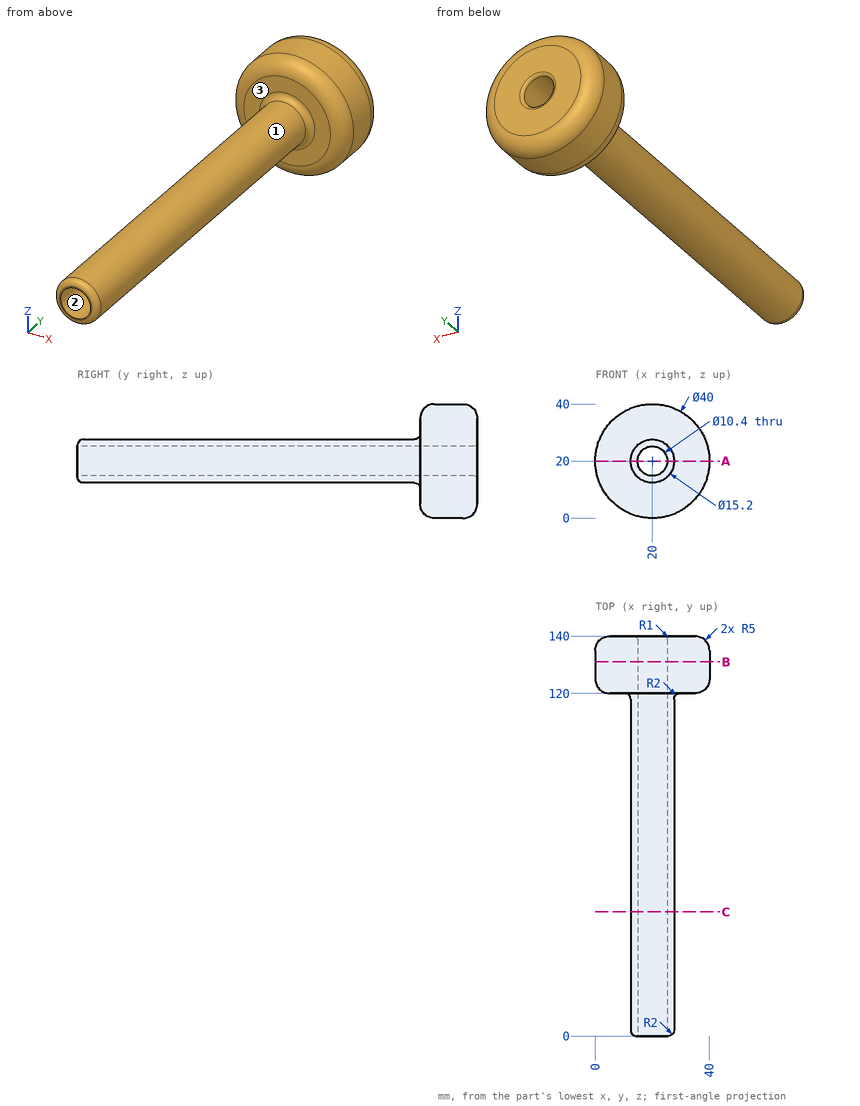
Design review of the part shown in the three views and the two pictorial views. Dimensions are in mm from the part's minimum x, y and z. Give positions to 0.01 mm unless a question says otherwise; leave off trailing zeros. Loops run counter-clockwise (first coordinate to the right, second up) from the corner with the lowest first, then second, coordinate; pieces in that order, holes last. Notation, with made-up numbers: (34, -40) -> (52, -40) arc R26 cw to (52, -1) -> close; hole circle Ø11 at (71.5, -24). An arc over 180 degrees is marked (long way). One line per item, written item: value.
Q1. We need section B-B on y = 131. Give the boundary of the cut face in (x, z).
Numbers:
outline: circle Ø40 at (20, 20); hole circle Ø10.4 at (20, 20)
Q2. For pin 1 Ø2 at (y, z) = (61, 20) entering from +X; pin 2 Ø15 at (x, z) = (18.5, 26.5) entering from -Y; pin 3 Ø5 at (y, z) = (42, 12.5) entering from -X; pin 4 Ø4 at (x, z) = (4.5, 7) entering from +Y, all flat-tipped, find the tip position at first contact; note any pin that passes through.
Numbers:
pin 1: stops at x = 27.6
pin 2: stops at y = 0
pin 3: stops at x = 14.28
pin 4: stops at y = 138.82
Q3. Draft analysis for pull direction X (two halves, no side actions). For the marked faces 1, 2 and 3, state which applies: pulls with the +X half, pulls with the -X half, needs draft (parallel to the pull), parting line crosses it, or undercut.
Numbers:
face 1: parting line crosses it
face 2: undercut
face 3: needs draft
Q4. For L1, parallel to X at y = 72, z = 20; L2, parallel to Z at x = 20.5, y = 116; L3, parallel to Y at x = 27.5, z = 6.5, list the stretches that pass through material, from the lowest coordinate up.
Numbers:
L1: x = 12.4 to 14.8, 25.2 to 27.6
L2: z = 12.42 to 14.82, 25.18 to 27.58
L3: y = 120.02 to 139.98
Q5. We need section C-C on y = 43.5. Give the boundary of the cut face in (x, z), and give its area (3 significant figures).
Numbers:
outline: circle Ø15.2 at (20, 20); hole circle Ø10.4 at (20, 20)
area: 96.5 mm^2
Q6. We need section A-A on z = 20. Give the boundary of the cut face in (x, y).
Numbers:
outline: (0, 125) arc R5 ccw to (5, 120) -> (10.4, 120) arc R2 cw to (12.4, 118) -> (12.4, 2) arc R2 ccw to (14.4, 0) -> (14.8, 0) -> (14.8, 139) arc R1 ccw to (13.8, 140) -> (5, 140) arc R5 ccw to (0, 135) -> close; (25.2, 0) -> (25.6, 0) arc R2 ccw to (27.6, 2) -> (27.6, 118) arc R2 cw to (29.6, 120) -> (35, 120) arc R5 ccw to (40, 125) -> (40, 135) arc R5 ccw to (35, 140) -> (26.2, 140) arc R1 ccw to (25.2, 139) -> close
